Could you check a few things on this model? Use its own coordinates, in mm. A direction names the side the tool comes from. Round coordinates to 2 decimals unless told otherwise and drop trailing zeros. Loops run counter-clockwise (first coordinate to the right, second up) from the corner with the lowest first, then second, coordinate; pieces in that order, holes last. Notation, with made-up numbers: (61, 55.25) -> (106, 55.25) arc R20 ccw to (106, 71.25) -> close; hole circle Ø8 at (60.5, -6.75). An arc over 180 degrees is marked (long way). Write each question's results on one line, items separated by ' | '.
from build123d import *

# Parameters (mm, degrees)
BOX250_W                  = 0.5
BOX250_H                  = 1
BOX250_DEPTH              = 15
BOX250_ROLL_ANGLE         = 46
BOX251_W                  = 0.5
BOX251_H                  = 1
BOX251_DEPTH              = 15
BOX251_ROLL_ANGLE         = -46
BOX249_W                  = 0.5
BOX249_H                  = 1
BOX249_DEPTH              = 11
FUSION026_PLACEMENT_ANGLE = -52.8


with BuildPart() as cubo250:
    # Box250 → Box250 (new body)
    with BuildSketch(Plane.XY):
        with Locations((0.25, 0.5)):
            Rectangle(BOX250_W, BOX250_H)
    extrude(amount=BOX250_DEPTH)


with BuildPart() as cubo250_1:
    # Box250 roll: moved
    add(cubo250.part.rotate(Axis((0, 0, 0), (1, 0, 0)), BOX250_ROLL_ANGLE))


with BuildPart() as cubo250_2:
    # Box250 placement: moved
    add(cubo250_1.part.moved(Location((0, 11, 0.5))))


with BuildPart() as cubo251:
    # Box251 → Box251 (new body)
    with BuildSketch(Plane.XY):
        with Locations((0.25, 0.5)):
            Rectangle(BOX251_W, BOX251_H)
    extrude(amount=BOX251_DEPTH)


with BuildPart() as cubo251_1:
    # Box251 roll: moved
    add(cubo251.part.rotate(Axis((0, 0, 0), (1, 0, 0)), BOX251_ROLL_ANGLE))


with BuildPart() as cubo251_2:
    # Box251 placement: moved
    add(cubo251_1.part.moved(Location((0, 0.4, 1.1))))


with BuildPart() as fusion026:
    # Box249 → Box249 (new body)
    with BuildSketch(Plane.XY.offset(0.5)):
        with Locations((0.25, 0.5)):
            Rectangle(BOX249_W, BOX249_H)
    extrude(amount=BOX249_DEPTH)

    # Fusion026: union Cubo250, Cubo251
    add(cubo250_2.part)
    add(cubo251_2.part)


with BuildPart() as fusion026_1:
    # Fusion026 placement: moved
    add(fusion026.part.moved(Location((-146.4, 182.7, 0))).rotate(Axis((-146.4, 182.7, 0), (0, 0, 1)), FUSION026_PLACEMENT_ANGLE))


solid = fusion026_1.part
1) If we mould it in two halves opening along Z, with no side actions, what happens to faces 1 (the flat face through (-142.336, 185.157, 6.801)), 2 (the flat face through (-143.4, 184.7, 2.8)), 3 (the flat face through (-138.85, 188.12, 3.54))? For each: released by +Z, released by -Z, zero draft, split by the parting line, or undercut.
Model answer:
face 1: zero draft | face 2: released by -Z | face 3: undercut
2) I want a section at B-B, the plane y = 187.75. Write out the boundary of the cut face in (x, z), plus the area to 3 significant figures.
Model answer:
outline: (-139.75, 3.06) -> (-138.92, 2.42) -> (-138.92, 3.81) -> (-139.75, 4.45) -> close; (-139.75, 7.39) -> (-138.92, 8.03) -> (-138.92, 9.42) -> (-139.75, 8.78) -> close | area: 2.30 mm2
3) I want a section at C-C, the plane x = -144.5. Write out the boundary of the cut face in (y, z).
Model answer:
outline: (183.51, 1.26) -> (184.14, 1.63) -> (184.14, 3.02) -> (183.51, 2.65) -> close; (183.51, 9.19) -> (184.14, 8.82) -> (184.14, 10.21) -> (183.51, 10.58) -> close
4) For faces 4 (the flat face through (-137.209, 189.367, 0.865)), 5 (the flat face through (-145.9, 182.8, 0.5)), 6 (the flat face through (-142.638, 185.555, 6.801)), 7 (the flat face through (-138.826, 188.139, 8.325)), 8 (the flat face through (-145.9, 182.7, 11.5)), which set-ups out of +Z, -Z, +X, -X, +Y, -Y let a thin tool reach every point of the face, with its end or its side?
Model answer:
face 4: -Z, +X, +Y | face 5: -Z, -X, -Y | face 6: +Z, -Z, -X, +Y | face 7: +X, +Y | face 8: +Z, -X, -Y
5) I want a section at A-A, the plane z = 9.75. Write out the boundary of the cut face in (x, y).
Model answer:
outline: (-146.4, 182.7) -> (-146.1, 182.3) -> (-145.3, 182.91) -> (-145.6, 183.3) -> close; (-145.27, 183.56) -> (-144.97, 183.16) -> (-143.82, 184.03) -> (-144.12, 184.43) -> close; (-138.95, 188.36) -> (-138.64, 187.96) -> (-137.5, 188.83) -> (-137.8, 189.23) -> close
6) I'm going to push flat-ended pins straight in: pin 1 (2 mm diameter, centred on x = -145, z = 7, fed in from +Y); pin 2 (3 mm diameter, centred on x = -143, z = 8.5, fed in from +Y); pin 3 (4 mm diameter, centred on y = 188.5, z = 5.5, fed in from +X). Where does each tip first touch, or does it pass through?
Model answer:
pin 1: stops at y = 183.3 | pin 2: stops at y = 185.96 | pin 3: stops at x = -138.74
7) I need wall thicknesses on line 1 (Z direction, x = -142.5, y = 185.5); line 2 (Y direction, x = -146, z = 4); line 3 (X direction, y = 188.25, z = 3.5). Which ranges of each line are inside material? Lowest first, please.
Model answer:
line 1: z = 3.96 to 5.35, 6.49 to 7.88 | line 2: y = 182.38 to 183 | line 3: x = -139.09 to -138.9
